Autodesk Inventor part; units mm, degrees
ref_plane "YZ Plane" through (0, 0, 0) normal (1, 0, 0) x (0, 1, 0)
ref_plane "XZ Plane" through (0, 0, 0) normal (0, 1, 0) x (-1, 0, 0)
ref_plane "XY Plane" through (0, 0, 0) normal (0, 0, 1) x (1, 0, 0)
sketch "Sketch1" plane through (0, 0, 0) normal (0, 0, 1) x (1, 0, 0)
  circle A0 centre (0, 0) radius 44.45
  line L0 (-44.45, 44.45) -> (44.45, 44.45)
  line L1 (44.45, 44.45) -> (44.45, -44.45)
  line L2 (44.45, -44.45) -> (-44.45, -44.45)
  line L3 (-44.45, -44.45) -> (-44.45, 44.45)
  dimension "d0" = 88.9
  dimension "d1" = 88.9
  dimension "d2" = 88.9
  dimension "d3" = 44.45
  dimension "d4" = 44.45
extrude "Extrusion1" add sketch "Sketch1" along normal blind 6.35
sketch "Sketch2" plane through (0, 0, 6.35) normal (0, 0, 1) x (1, 0, 0)
  circle A0 centre (0, 0) radius 46.0375
  circle A1 centre (0, 0) radius 44.45
  line L0 (0, 39.444) -> (19.722, 34.1595)
  line L1 (19.722, 34.1595) -> (34.1595, 19.722)
  line L2 (34.1595, 19.722) -> (39.444, 0)
  line L3 (39.444, 0) -> (34.1595, -19.722)
  line L4 (34.1595, -19.722) -> (19.722, -34.1595)
  line L5 (19.722, -34.1595) -> (0, -39.444)
  line L6 (0, -39.444) -> (-19.722, -34.1595)
  line L7 (-19.722, -34.1595) -> (-34.1595, -19.722)
  line L8 (-34.1595, -19.722) -> (-39.444, 0)
  line L9 (-39.444, 0) -> (-34.1595, 19.722)
  line L10 (-34.1595, 19.722) -> (-19.722, 34.1595)
  line L11 (-19.722, 34.1595) -> (0, 39.444)
  dimension "d8" = 1.5875
  dimension "d25" = 76.2
  dimension "d46" = 88.9
extrude "Extrusion2" add sketch "Sketch2" along normal blind 63.5 contours A1
sketch "Sketch3" plane through (0, 0, 6.35) normal (0, 0, 1) x (1, 0, 0)
  circle A0 centre (0, 0) radius 14.2875
  dimension "d11" = 28.575
extrude "Extrusion3" cut sketch "Sketch3" against normal blind 38.1
sketch "Sketch4" plane through (0, 0, 6.35) normal (0, 0, 1) x (1, 0, 0)
  circle A0 centre (0, 0) radius 14.2875
  circle A1 centre (0, 0) radius 19.05
  dimension "d14" = 38.1
extrude "Extrusion4" add sketch "Sketch4" along normal blind 34.925
sketch "Sketch6" plane through (0, 0, 6.35) normal (0, 0, 1) x (1, 0, 0)
  circle A0 centre (31.75, 0) radius 6.35
  point P0 (0, 0)
  dimension "d21" = 12.7
  dimension "d22" = 31.75
extrude "Extrusion6" cut sketch "Sketch6" against normal blind 25.4
sketch "Sketch7" plane through (0, 0, 6.35) normal (0, 0, 1) x (1, 0, 0)
  line L0 (0, 44.45) -> (-44.45, 44.45)
  line L1 (-44.45, 44.45) -> (-44.45, 0)
  line L2 (0, -44.45) -> (44.45, -44.45)
  line L3 (44.45, 0) -> (44.45, 44.45)
  arc A0 (44.45, 0) -> (0, 44.45) centre (0, 0) ccw
  line L4 (44.45, -44.45) -> (44.45, 44.45)
  arc A1 (0, 44.45) -> (-44.45, 0) centre (0, 0) ccw
  arc A2 (-44.45, 0) -> (0, -44.45) centre (0, 0) ccw
  line L5 (-44.45, 0) -> (-44.45, -44.45)
  line L6 (44.45, 44.45) -> (0, 44.45)
  arc A3 (0, -44.45) -> (44.45, 0) centre (0, 0) ccw
  line L7 (44.45, -44.45) -> (44.45, 0)
  line L8 (-44.45, -44.45) -> (0, -44.45)
  line L9 (-44.45, 0) -> (-44.45, -44.45)
  line L10 (-44.45, -44.45) -> (0, -44.45)
  line L11 (44.45, -44.45) -> (-44.45, -44.45)
  line L12 (0, -44.45) -> (44.45, -44.45)
  line L13 (44.45, -44.45) -> (44.45, 0)
  arc A4 (-44.45, 0) -> (0, -44.45) centre (0, 0) ccw
  arc A5 (0, -44.45) -> (44.45, 0) centre (0, 0) ccw
  point P0 (-44.4261, -1.4578)
  point P1 (44.4261, -1.4578)
extrude "Extrusion7" cut sketch "Sketch7" against normal blind 25.4 contours L4 L2 A3 | A2 L8 L5
sketch "Sketch8" plane through (0, 0, 0) normal (0, 1, 0) x (-1, 0, 0)
  line L0 (44.45, 0) -> (44.45, 69.85)
  arc A0 (44.45, 56.8325) -> (44.45, 51.1175) centre (45.974, 53.975) ccw
  arc A1 (44.45, 21.9075) -> (44.45, 16.1925) centre (45.974, 19.05) ccw
  line L1 (44.45, 69.85) -> (-44.45, 69.85)
  line L2 (0, -13.97) -> (0, 83.82)
  arc A2 (44.2147, 16.3311) -> (44.45, 21.9075) centre (45.974, 19.05) ccw
  point P0 (0, 0)
  dimension "d28" = 3.2385
  dimension "d31" = 19.05
  dimension "d32" = 15.875
  dimension "d45" = 1.7145
revolve "Revolution1" cut sketch "Sketch8" angle 360 about axis through (0, 0, -10) along (0, 0, 1) contours A1 L0 | A0 L0
sketch "Sketch9" plane through (0, 0, 6.35) normal (0, 0, 1) x (1, 0, 0)
  circle A0 centre (31.75, 0) radius 6.35
  circle A1 centre (0, 0) radius 19.05
  line L0 (34.1595, 19.722) -> (19.722, 34.1595)
  line L1 (19.722, 34.1595) -> (0, 39.444)
  line L2 (0, 39.444) -> (-19.722, 34.1595)
  line L3 (-19.722, 34.1595) -> (-34.1595, 19.722)
  line L4 (-34.1595, 19.722) -> (-39.444, 0)
  line L5 (-39.444, 0) -> (-34.1595, -19.722)
  line L6 (-34.1595, -19.722) -> (-19.722, -34.1595)
  line L7 (-19.722, -34.1595) -> (0, -39.444)
  line L8 (0, -39.444) -> (19.722, -34.1595)
  line L9 (19.722, -34.1595) -> (34.1595, -19.722)
  line L10 (34.1595, -19.722) -> (39.444, 0)
  line L11 (39.444, 0) -> (34.1595, 19.722)
  circle A2 centre (0, -31.75) radius 4.826
  dimension "d35" = 9.652
  dimension "d36" = 31.75
  dimension "d37" = 31.75
extrude "Extrusion8" cut sketch "Sketch9" against normal blind 25.4 contours A2
sketch "Sketch10" plane through (0, 0, 6.35) normal (0, 0, 1) x (1, 0, 0)
  circle A0 centre (0, -31.75) radius 4.826
  circle A1 centre (31.75, 0) radius 6.35
  circle A2 centre (0, 0) radius 19.05
  line L0 (34.1595, 19.722) -> (19.722, 34.1595)
  line L1 (19.722, 34.1595) -> (0, 39.444)
  line L2 (0, 39.444) -> (-19.722, 34.1595)
  line L3 (-19.722, 34.1595) -> (-34.1595, 19.722)
  line L4 (-34.1595, 19.722) -> (-39.444, 0)
  line L5 (-39.444, 0) -> (-34.1595, -19.722)
  line L6 (-34.1595, -19.722) -> (-19.722, -34.1595)
  line L7 (-19.722, -34.1595) -> (0, -39.444)
  line L8 (0, -39.444) -> (19.722, -34.1595)
  line L9 (19.722, -34.1595) -> (34.1595, -19.722)
  line L10 (34.1595, -19.722) -> (39.444, 0)
  line L11 (39.444, 0) -> (34.1595, 19.722)
  arc A3 (7.6781, -37.3867) -> (-7.6781, -37.3867) centre (0, -31.75) ccw
  dimension "d40" = 19.05
extrude "Extrusion9" cut sketch "Sketch10" against normal blind 3.175 contours L8 L7 A3
sketch "Sketch11" plane through (0, 0, 0) normal (0, 1, 0) x (-1, 0, 0)
  line L0 (-19.05, 6.35) -> (-19.05, 41.275)
  line L1 (-19.05, 38.1) -> (-26.605, 25.4)
  line L2 (-26.605, 25.4) -> (-23.8011, 25.4)
  line L3 (44.45, 21.9075) -> (-44.45, 21.9075)
  line L4 (-23.8011, 25.4) -> (-17.684, 35.6829)
  point P0 (0, 0)
  dimension "d43" = 25.4
  dimension "d44" = 12.7
sketch "Sketch12" plane through (-44.45, 44.45, 0) normal (0, 1, 0) x (1, 0, 0)
  line L0 (0, 0) -> (88.9, 0)
  line L1 (0, 0) -> (0, -6.35)
  line L2 (44.45, -6.35) -> (0, -6.35)
  line L3 (88.9, -6.35) -> (44.45, -6.35)
  line L4 (88.9, 0) -> (88.9, -6.35)
  point P0 (44.45, 0)
extrude "Extrusion10" add sketch "Sketch12" along normal blind 12.7
sketch "Sketch13" plane through (0, 0, 0) normal (0, 0, -1) x (-1, 0, 0)
  circle A0 centre (0, 0) radius 44.45
  arc A1 (44.45, 0) -> (-44.45, 0) centre (0, 0) ccw
  line L0 (-7.4513, 43.821) -> (0.0223, 44.45)
  line L1 (0.0223, 44.45) -> (0.2739, 41.4606)
  line L2 (0.2739, 41.4606) -> (-7.1997, 40.8316)
  line L3 (-7.1997, 40.8316) -> (-7.4513, 43.821)
  line L4 (4.1443, 44.2564) -> (11.526, 42.9296)
  line L5 (11.526, 42.9296) -> (10.9953, 39.9769)
  line L6 (10.9953, 39.9769) -> (3.6136, 41.3037)
  line L7 (3.6136, 41.3037) -> (4.1443, 44.2564)
  line L8 (0, 0) -> (0, 64.8467) construction
  line L9 (0, 0) -> (-11.2605, 63.8615) construction
  line L10 (0, 0) -> (-22.1789, 60.936) construction
  line L11 (0, 0) -> (-32.4234, 56.1589) construction
  line L12 (0, 0) -> (-41.6827, 49.6755) construction
  line L13 (0, 0) -> (-49.6755, 41.6827) construction
  line L14 (0, 0) -> (-56.1589, 32.4234) construction
  line L15 (0, 0) -> (-60.936, 22.1789) construction
  line L16 (0, 0) -> (-63.8615, 11.2605) construction
  line L17 (0, 0) -> (-64.8467, 0) construction
  line L18 (0, 0) -> (-63.8615, -11.2605) construction
  line L19 (0, 0) -> (-60.936, -22.1789) construction
  line L20 (0, 0) -> (-56.1589, -32.4234) construction
  line L21 (0, 0) -> (-49.6755, -41.6827) construction
  line L22 (0, 0) -> (-41.6827, -49.6755) construction
  line L23 (0, 0) -> (-32.4234, -56.1589) construction
  line L24 (0, 0) -> (-22.1789, -60.936) construction
  line L25 (0, 0) -> (-11.2605, -63.8615) construction
  line L26 (0, 0) -> (0, -64.8467) construction
  line L27 (0, 0) -> (11.2605, -63.8615) construction
  line L28 (0, 0) -> (22.1789, -60.936) construction
  line L29 (0, 0) -> (32.4234, -56.1589) construction
  line L30 (0, 0) -> (41.6827, -49.6755) construction
  line L31 (0, 0) -> (49.6755, -41.6827) construction
  line L32 (0, 0) -> (56.1589, -32.4234) construction
  line L33 (0, 0) -> (60.936, -22.1789) construction
  line L34 (0, 0) -> (63.8615, -11.2605) construction
  line L35 (0, 0) -> (64.8467, 0) construction
  line L36 (0, 0) -> (63.8615, 11.2605) construction
  line L37 (0, 0) -> (60.936, 22.1789) construction
  line L38 (0, 0) -> (56.1589, 32.4234) construction
  line L39 (0, 0) -> (49.6755, 41.6827) construction
  line L40 (0, 0) -> (41.6827, 49.6755) construction
  line L41 (0, 0) -> (32.4234, 56.1589) construction
  line L42 (0, 0) -> (22.1789, 60.936) construction
  line L43 (0, 0) -> (11.2605, 63.8615) construction
  point P0 (0, -44.45)
  dimension "d53" = 7.5
  dimension "d54" = 3
  dimension "d55" = 3
  dimension "d56" = 7.5
  dimension "d59" = 360
  dimension "d61" = 15
extrude "Extrusion11" cut sketch "Sketch13" against normal blind 13.35 contours L4 A0 | L5 L6 L7 L4 | A0 L0 | L0 L1 L2 L3
sketch "Sketch14" plane through (0, 0, 0) normal (0, 0, -1) x (-1, 0, 0)
  circle A0 centre (10.2313, 30.0563) radius 2.7115
  circle A1 centre (-15.0804, 27.94) radius 2.7115
  circle A2 centre (-22.5999, -22.3004) radius 2.7115
  circle A3 centre (0, 0) radius 14.2875
  dimension "d64" = 5.4229
  dimension "d71" = 31.75
  dimension "d72" = 31.75
  dimension "d73" = 31.75
  dimension "d74" = 25.4
  dimension "d75" = 50.8
  dimension "d76" = 27.94
extrude "Extrusion12" cut sketch "Sketch14" against normal blind 25.4 contours A0 | A1 | A2
sketch "Sketch15" plane through (0, 0, 0) normal (0, 0, -1) x (-1, 0, 0)
  circle A0 centre (-31.75, 7.75) radius 1.004
  circle A1 centre (-31.75, -7.75) radius 1.004
  circle A2 centre (-31.75, 0) radius 6.35
  point P0 (0, 0)
  dimension "d77" = 7.75
  dimension "d78" = 15.5
  dimension "d79" = 2.008
extrude "Extrusion13" cut sketch "Sketch15" against normal blind 25.4 contours A0 | A1
equation "\"d55\" = d54"
equation "\"d56\" = d53"
equation "\"d77\" = 0.5 * d78"
properties part number "mounting plate"
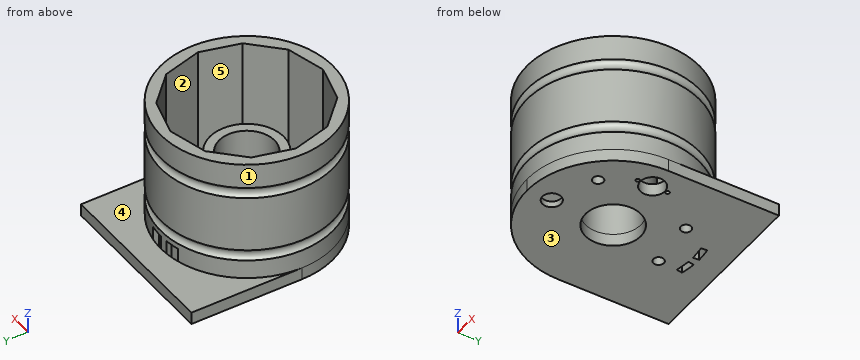
The listing builds one solid part. Answer for the finished solid, in the listing's coordinates (mm). Face numbers are marked on the shaded views. A direction names the side the tool comes from. Give positions to 0.01 mm unless a question says otherwise; leave off trailing zeros. Write each loop counter-clockwise with the first axis right and the second up, starting at its lowest first coordinate (ties: lowest second). Pieces come first, ordered by that corner, then holes.
1) A tool of negligible diameter and unlimited length cuts with its end or side. For the marked faces 4 and 5, from which of +Z, -Z, +X, -X, +Y, -Y can it reach the whole face along a straight path? Write none if from no direction.
2) For a pull along X with two mould halves and no side action, classify the marked faces 1, 2 and 3 as pulls with the +X half, pulls with the -X half, needs draft (parallel to the pull), parting line crosses it, or undercut.
3) Section B-B (z = 63.5) is taken. Write down the section's boundary in (x, y), and give its area (3 significant figures).
4) Find the intervals of material crossed by L1, parallel to Y at x = 0, z = 27; L2, parallel to X at y = -7, z = 3; L3, parallel to Y at x = 16, z = 29, in increasing order.
5) Section A-A (z = 11) is taken. Count the separate pieces of the cut face and the enclosed holes in it, and give its area (3 significant figures).
6) Given P1, Ø3, axis at x = 5, z = 57, coming from the +Y side; P2, Ø2.5, axis at x = 31.75, y = -7.75, coming from the +Z side; P3, Ø1, axis at y = 34, z = 13, coming from the -X side; P4, Ø7, axis at x = 15.08, y = 27.94, coming from the -Z side, each flat-ended and moving along its own axis, determine where each tip first touches the part or whether it passes through.
Response:
1. face 4: +Z, +Y
1. face 5: +Z
2. face 1: parting line crosses it
2. face 2: undercut
2. face 3: needs draft
3. outline: circle Ø88.9 at (0, 0); hole (-39.44, 0) - (-34.16, -19.72) - (-19.72, -34.16) - (0, -39.44) - (19.72, -34.16) - (34.16, -19.72) - (39.44, 0) - (34.16, 19.72) - (19.72, 34.16) - (0, 39.44) - (-19.72, 34.16) - (-34.16, 19.72) - close
3. area: 1,540 mm2
4. L1: y = -44.45 to -39.44, -19.05 to -14.29, 14.29 to 19.05, 39.44 to 44.45
4. L2: x = -43.9 to -12.46, 12.46 to 31.08, 32.42 to 43.9
4. L3: y = -41.47 to -35.16, -10.34 to 10.34, 35.16 to 41.47
5. separate pieces: 2
5. enclosed holes: 2
5. area: 1,990 mm2
6. P1: stops at y = 44.31
6. P2: stops at z = 6.35
6. P3: stops at x = -29.22
6. P4: stops at z = 0
